Check sheet for the drawn part. Datum: minimum x, y, z corner. Units: mm. A direction names the side the tool comes from. Round coordinates to 2 decimals unless told otherwise and drop trailing zeros. Loops run counter-clockwise (first coordinate to the right, second up) from the corner with the lowest first, then second, coordinate; pieces in that order, holes last. Notation, with made-up numbers: (-19.5, -37) -> (23.5, -37) arc R24 ccw to (23.5, -10) -> close; hole circle Ø10 at (53.5, 51). An arc over 180 degrees is marked (long way). Write item = value, one per line. Start each with the question number.
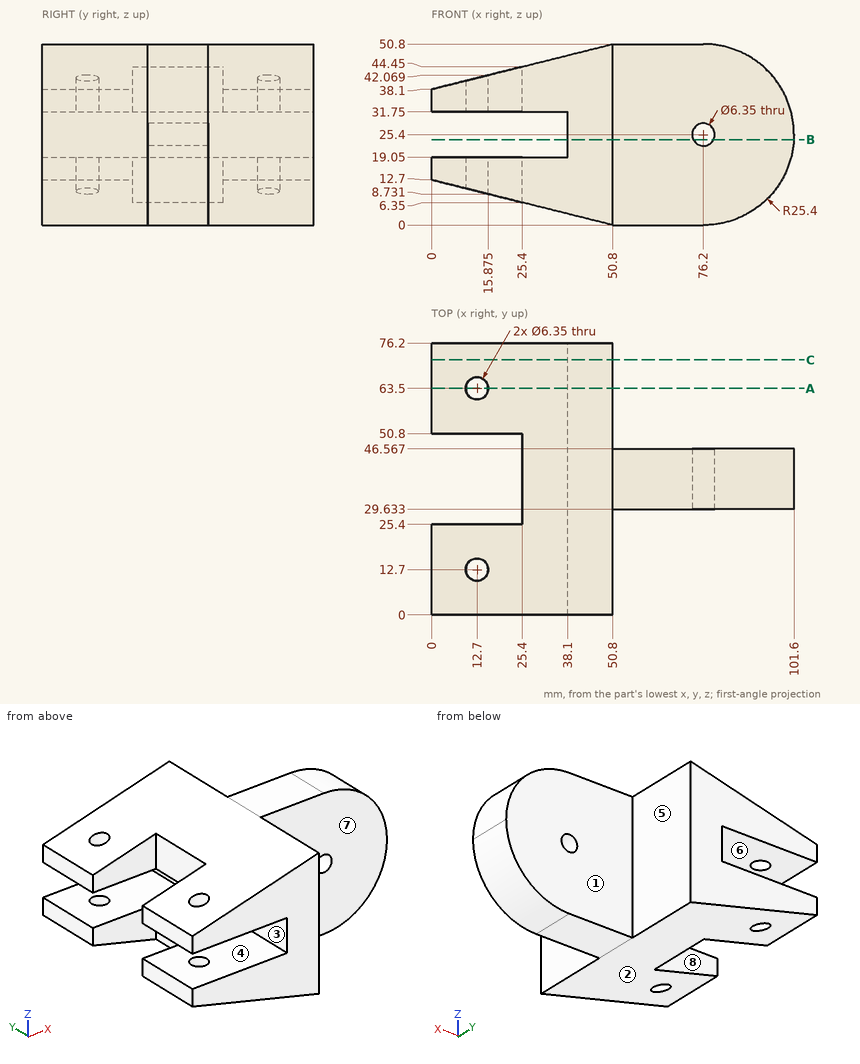
(1) Section check A-A on y = 63.5. Give the number of separate pieces and of enclosed holes in the cut face, then the cut area to 3 significant figures.
(2) Access from +Z, -Z, +X, -X, +Y, -Y to the whole of each face (thin tool, end or side, straight path). Record for the marked faces 5, 6, 7 and 8.
(3) Section check B-B on z = 24. Enter the section's corners in (x, y).
(4) Scan lines: line 1 (Y direction, x = 12.7, z = 34.75) (1 decimal); line 2 (X direction, y = 12.7, z = 13.25) (1 decimal); line 3 (Y direction, x = 12, z = 15). Record each from-to range of solid material in increasing order. Write a range as [from, to].
(5) Depth check by flat-ended pin: pin 1 Ø5 at (x, y) = (12.7, 63.5) entering from -Z; pin 2 Ø4 at (x, y) = (82, 36) entering from +Z; pin 3 Ø15 at (y, z) = (55.5, 32.5) entering from +X; pin 4 Ø7.5 at (x, y) = (12.7, 12.7) entering from -Z. Enter the tip coordinate at first touch or a pass-through.
(6) Draft check along Z on the marked faces 1, 2, 3 and 4. Enter one of: +Z half, -Z half, draft (parallel to the pull), parting line (faces both ways), or undercut.
(7) Section check C-C on y = 71.5. Enter the section's corners in (x, z).
Computed values:
q1.separate_pieces = 3
q1.enclosed_holes = 0
q1.area = 1,330 mm²
q2.face_5 = +Z, -Z, +X, +Y
q2.face_6 = -X, +Y, -Y
q2.face_7 = +Z, -Z, +X, -Y
q2.face_8 = +Z, -Z, -X
q3.outline = (38.1, 0) -> (50.8, 0) -> (50.8, 29.63) -> (73.35, 29.63) -> (73.35, 46.57) -> (50.8, 46.57) -> (50.8, 76.2) -> (38.1, 76.2) -> close; (79.05, 29.63) -> (101.56, 29.63) -> (101.56, 46.57) -> (79.05, 46.57) -> close
q4.line_1 = [0, 9.5], [15.9, 25.4], [50.8, 60.3], [66.7, 76.2]
q4.line_2 = [0, 9.5], [15.9, 50.8]
q4.line_3 = [0, 9.6], [15.8, 25.4], [50.8, 60.4], [66.6, 76.2]
q5.pin_1 = through
q5.pin_2 = 50.51
q5.pin_3 = 50.8
q5.pin_4 = 8.59
q6.face_1 = draft
q6.face_2 = -Z half
q6.face_3 = undercut
q6.face_4 = undercut
q7.outline = (0, 12.7) -> (50.8, 0) -> (50.8, 50.8) -> (0, 38.1) -> (0, 31.75) -> (38.1, 31.75) -> (38.1, 19.05) -> (0, 19.05) -> close
